```python
from build123d import *

# Parameters (mm, degrees)
BOSS_EXTRUDE1_DEPTH = 1
SKETCH2_R           = 1.5
BOSS_EXTRUDE2_DEPTH = 6


with BuildPart() as part:
    # Sketch1 → Boss-Extrude1 (new body)
    with BuildSketch(Plane(origin=(0, 0, 0), x_dir=(1, 0, 0), z_dir=(0, 1, 0))):
        with BuildLine():
            Line((0.038153439, 3.037815087), (0.816252158, 3.809013473))
            ThreePointArc((0.816252158, 3.809013473), (1.082123997, 3.875868882), (1.274025664, 3.680085251))
            Line((1.274025664, 3.680085251), (1.551949391, 2.611748318))
            Line((1.551949391, 2.611748318), (2.611401842, 2.890576352))
            ThreePointArc((2.611401842, 2.890576352), (2.875081312, 2.815538915), (2.943381216, 2.550034483))
            Line((2.943381216, 2.550034483), (2.649901757, 1.485865696))
            Line((2.649901757, 1.485865696), (3.70682851, 1.197611631))
            ThreePointArc((3.70682851, 1.197611631), (3.897662912, 1.00078757), (3.824060148, 0.736704035))
            Line((3.824060148, 0.736704035), (3.037815087, -0.038153439))
            Line((3.037815087, -0.038153439), (3.809013473, -0.816252158))
            ThreePointArc((3.809013473, -0.816252158), (3.875868882, -1.082123997), (3.680085251, -1.274025664))
            Line((3.680085251, -1.274025664), (2.611748318, -1.551949391))
            Line((2.611748318, -1.551949391), (2.890576352, -2.611401842))
            ThreePointArc((2.890576352, -2.611401842), (2.815538915, -2.875081312), (2.550034483, -2.943381216))
            Line((2.550034483, -2.943381216), (1.485865696, -2.649901757))
            Line((1.485865696, -2.649901757), (1.197611631, -3.70682851))
            ThreePointArc((1.197611631, -3.70682851), (1.00078757, -3.897662912), (0.736704035, -3.824060148))
            Line((0.736704035, -3.824060148), (-0.038153439, -3.037815087))
            Line((-0.038153439, -3.037815087), (-0.816252158, -3.809013473))
            ThreePointArc((-0.816252158, -3.809013473), (-1.082123997, -3.875868882), (-1.274025664, -3.680085251))
            Line((-1.274025664, -3.680085251), (-1.551949391, -2.611748318))
            Line((-1.551949391, -2.611748318), (-2.611401842, -2.890576352))
            ThreePointArc((-2.611401842, -2.890576352), (-2.875081312, -2.815538915), (-2.943381216, -2.550034483))
            Line((-2.943381216, -2.550034483), (-2.649901757, -1.485865696))
            Line((-2.649901757, -1.485865696), (-3.70682851, -1.197611631))
            ThreePointArc((-3.70682851, -1.197611631), (-3.897662912, -1.00078757), (-3.824060148, -0.736704035))
            Line((-3.824060148, -0.736704035), (-3.037815087, 0.038153439))
            Line((-3.037815087, 0.038153439), (-3.809013473, 0.816252158))
            ThreePointArc((-3.809013473, 0.816252158), (-3.875868882, 1.082123997), (-3.680085251, 1.274025664))
            Line((-3.680085251, 1.274025664), (-2.611748318, 1.551949391))
            Line((-2.611748318, 1.551949391), (-2.890576352, 2.611401842))
            ThreePointArc((-2.890576352, 2.611401842), (-2.815538915, 2.875081312), (-2.550034483, 2.943381216))
            Line((-2.550034483, 2.943381216), (-1.485865696, 2.649901757))
            Line((-1.485865696, 2.649901757), (-1.197611631, 3.70682851))
            ThreePointArc((-1.197611631, 3.70682851), (-1.00078757, 3.897662912), (-0.736704035, 3.824060148))
            Line((-0.736704035, 3.824060148), (0.038153439, 3.037815087))
        make_face()
    extrude(amount=BOSS_EXTRUDE1_DEPTH)

    # Sketch2 → Boss-Extrude2 (add)
    with BuildSketch(Plane.XZ):
        Circle(SKETCH2_R)
    extrude(amount=BOSS_EXTRUDE2_DEPTH)


solid = part.part
```
Could you check a few things on this model? Use its own coordinates, in mm. A direction names the side the tool comes from. Round coordinates to 2 decimals unless told otherwise and drop trailing zeros. Loops run counter-clockwise (first coordinate to the right, second up) from the corner with the lowest first, then second, coordinate; pieces in that order, holes last. Notation, with made-up numbers: (51, 73.5) - (91, 73.5) arc R13 cw to (91, 87.5) - close; hole circle Ø4 at (45, -24.5). An arc over 180 degrees is marked (long way). Answer as CSV lines item,"result".
1. I want a section at A-A on y = -2. List the corners of the cut face in (x, z) for me, then the cut area to 3 significant figures.
Filled in:
outline,"circle Ø3 at (0, 0)"
area,"7.07 mm^2"
2. On a 3-axis mill with a long thin cutter (end or side, diameter ignored), from which of +Z, -Z, +X, -X, +Y, -Y can I reach the whole of each face in a straight line? I mean faces 1 (the face through (-1.5, -2.96, 0.07)), 2 (the face through (-1.344, 0.493, -3.171)), 3 (the face through (-1.4, 0.5, 3.2)). Say none if no direction works.
Filled in:
face 1,"-Y"
face 2,"-Z, +Y, -Y"
face 3,"+Z, +Y, -Y"
3. I want a section at C-C on z = 2.25. List the corners of the cut face in (x, y) for me.
Filled in:
outline,"(-2.86, 0) - (2.8, 0) - (2.8, 1) - (-2.86, 1) - close"
4. We'd pull the mould along Z, two halves only. Please class faces 4 (the face through (-3.171, 0.493, 1.344)), 5 (the face through (0, 1, 0)), 6 (the face through (-2.07, 0.49, 2.75)): +Z half, -Z half, draft (parallel to the pull), parting line (faces both ways), or undercut.
Filled in:
face 4,"undercut"
face 5,"draft"
face 6,"+Z half"
5. Please list where these lines run through material, in increasing order: line 1 along Y through (x, z) = (3.25, -1); line 2 along Z through (x, y) = (0, -5); line 3 along X through (y, z) = (-2, 1). Write a range as [from, to].
Filled in:
line 1,"y = [0, 1]"
line 2,"z = [-1.5, 1.5]"
line 3,"x = [-1.12, 1.12]"
6. I want a section at B-B on z = 0.5. List the corners of the cut face in (x, y) for me, then the cut area to 4 significant figures.
Filled in:
outline,"(-3.58, 0) - (-1.41, 0) - (-1.41, -6) - (1.41, -6) - (1.41, 0) - (3.5, 0) - (3.5, 1) - (-3.58, 1) - close"
area,"24.05 mm^2"
